The listing builds one solid part. Answer for the finished solid, in the listing's coordinates (mm). Coordinates: 2 decimals unless noted, no trailing zeros. Write each loop counter-clockwise with the first axis right and the second up, starting at its lowest first coordinate (ties: lowest second). Pieces come first, ordered by that corner, then holes.
Autodesk Inventor part; units mm, degrees
ref_plane "YZ Plane" through (0, 0, 0) normal (1, 0, 0) x (0, 1, 0)
ref_plane "XZ Plane" through (0, 0, 0) normal (0, 1, 0) x (-1, 0, 0)
ref_plane "XY Plane" through (0, 0, 0) normal (0, 0, 1) x (1, 0, 0)
sketch "草圖1" plane through (0, 0, 0) normal (0, 0, 1) x (1, 0, 0)
  line L0 (0, -5) -> (0, 5) construction
  line L1 (2, -5) -> (2, 5)
  line L2 (-2, 5) -> (-2, -5)
  arc A0 (-2, -5) -> (2, -5) centre (0, -5) ccw
  arc A1 (2, 5) -> (-2, 5) centre (0, 5) ccw
  point P0 (0, 0)
  dimension "d0" = 10
  dimension "d21" = 4
extrude "擠出1" add sketch "草圖1" along normal mid plane 1
sketch "草圖2" plane through (0, 0, 0) normal (0, 0, 1) x (1, 0, 0)
  arc A0 (-2, -5) -> (2, -5) centre (0, -5) ccw
  circle A1 centre (0, -5) radius 0.75
  point P0 (0, 0)
  dimension "d3" = 1.5
extrude "擠出2" add sketch "草圖2" along normal mid plane 3
sketch "草圖3" plane through (0, 0, 0) normal (0, 0, 1) x (1, 0, 0)
  arc A0 (2, 5) -> (-2, 5) centre (0, 5) ccw
  circle A1 centre (0, 5) radius 0.75
  point P0 (0, 0)
  dimension "d6" = 1.5
extrude "擠出3" add sketch "草圖3" along normal mid plane 3
sketch "草圖4" plane through (2, -5, 0.5) normal (1, 0, 0) x (0, 0, -1)
  line L0 (0, 0) -> (0, -2)
  line L1 (0, -2) -> (-2.346, -2)
  line L2 (-2.346, -2) -> (-2.346, 2.4059)
  line L3 (-2.346, 2.4059) -> (0, 2.4059)
  line L4 (0, 2.4059) -> (0, -2)
  point P0 (0.5, 5)
extrude "擠出4" cut sketch "草圖4" against normal blind 10
sketch "草圖5" plane through (0, 0, -0.5) normal (0, 0, -1) x (-1, 0, 0)
  circle A0 centre (0, 5) radius 0.75
  point P0 (0, 0)
extrude "擠出5" cut sketch "草圖5" along normal blind 10
sketch "草圖7" plane through (0, 5, 1.5) normal (0, 0, 1) x (1, 0, 0)
  circle A0 centre (0, 0) radius 0.75
  circle A1 centre (0, 0) radius 0.75
  circle A2 centre (0, -10) radius 0.75
  point P0 (0, -5)
extrude "擠出7" cut sketch "草圖7" against normal blind 10
sketch "草圖8" plane through (0, 0, 0.5) normal (0, 0, 1) x (1, 0, 0)
  circle A0 centre (0, 5) radius 0.75
  circle A1 centre (0, 5) radius 1
  circle A2 centre (0, -5) radius 0.75
  circle A3 centre (0, -5) radius 1
  point P0 (0, 0)
  dimension "d17" = 2
  dimension "d18" = 2
extrude "擠出8" cut sketch "草圖8" against normal blind 10
properties part number "圓盤"
(1) Find the intervals of material crossed by probe 1 along Y at (x, z) = (0, -0.2); probe 2 along Y at (x, z) = (0.65, -0.3); probe 3 along X at (y, z) = (-5.75, 0.05), in increasing order.
(2) Section A-A, the plane x = 0 is taken. Write down the section's boundary in (y, z).
(3) For a pull along X with two mould halves and no side action, classify faces 1 (the cylindrical face through (0, -7, 0)), 2 (the flat face through (0, 0, -0.5)), 3 (the cylindrical face through (0, 6, 0)) as pulls with the +X half, pulls with the -X half, needs draft (parallel to the pull), parting line crosses it, or undercut.
(4) Section B-B, the plane z = 0.2 is taken. Write down the section's boundary in (x, y).
(5) Section C-C, the plane y = 5.25 is taken. Write down the section's boundary in (x, z), plus the area to 3 significant figures.
(6) Section D-D, the plane x = -1.7 is taken. Write down the section's boundary in (y, z), plus the area to 3 significant figures.
Solution:
1. probe 1: y = -7 to -6, -4 to 4, 6 to 7
1. probe 2: y = -6.89 to -5.76, -4.24 to 4.24, 5.76 to 6.89
1. probe 3: x = -1.85 to -0.66, 0.66 to 1.85
2. outline: (-7, -0.5) - (-6, -0.5) - (-6, 0.5) - (-7, 0.5) - close; (-4, -0.5) - (4, -0.5) - (4, 0.5) - (-4, 0.5) - close; (6, -0.5) - (7, -0.5) - (7, 0.5) - (6, 0.5) - close
3. face 1: parting line crosses it
3. face 2: needs draft
3. face 3: undercut
4. outline: (-2, -5) arc R2 ccw to (2, -5) - (2, 5) arc R2 ccw to (-2, 5) - close; hole circle Ø2 at (0, -5); hole circle Ø2 at (0, 5)
5. outline: (-1.98, -0.5) - (-0.97, -0.5) - (-0.97, 0.5) - (-1.98, 0.5) - close; (0.97, -0.5) - (1.98, -0.5) - (1.98, 0.5) - (0.97, 0.5) - close
5. area: 2.03 mm2
6. outline: (-6.05, -0.5) - (6.05, -0.5) - (6.05, 0.5) - (-6.05, 0.5) - close
6. area: 12.1 mm2
